Job drawing, mm, ordinate dimensions from the low corner. One solid piece. Coordinates: 2 decimals unless noted, no trailing zeros. Order: outer loops, then holes, each group sorted by start corner. A loop starts at its lowest first (then second) coordinate and runs counter-clockwise, first axis right, second up. Notation, with made-up numbers: (81, 69) - (127, 69) arc R19 ccw to (127, 89) - close; hole circle Ø1 at (35, 65.25). An arc over 180 degrees is marked (long way). Return JSON: item names as keys, results as strings.
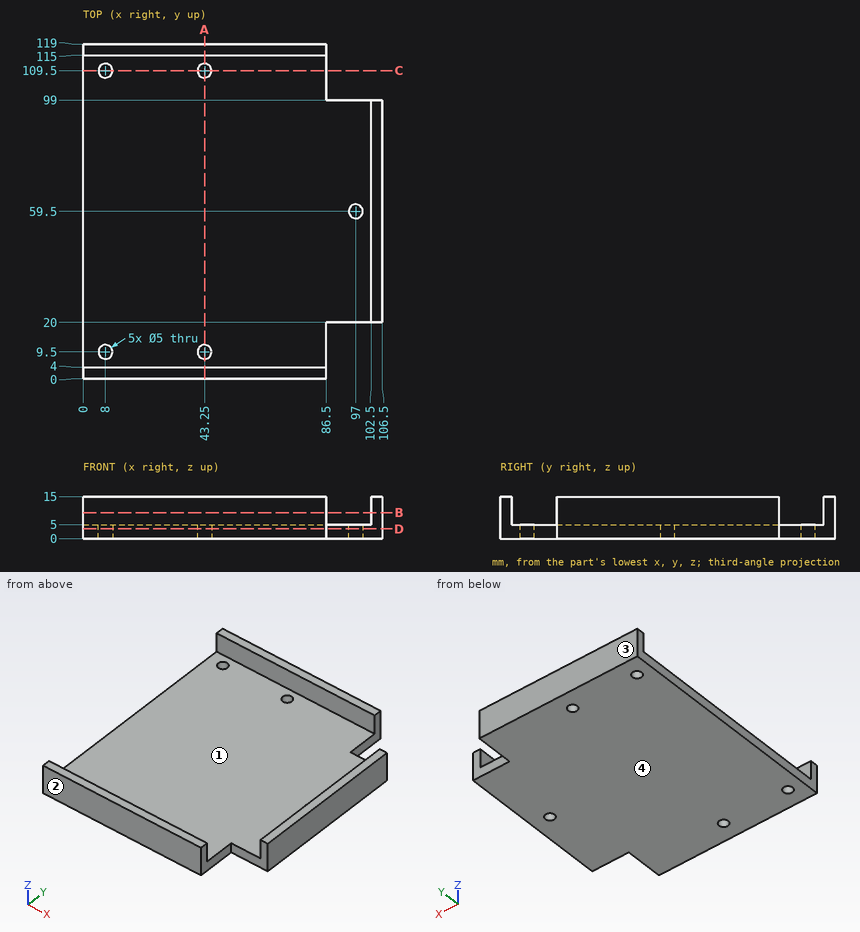
1. Cut at B-B on z = 9.25. Give the cut face in (x, y), plus the area to 3 significant figures.
Check values:
{"outline": "(0, 0) - (86.5, 0) - (86.5, 4) - (0, 4) - close; (0, 115) - (86.5, 115) - (86.5, 119) - (0, 119) - close; (102.5, 20) - (106.5, 20) - (106.5, 99) - (102.5, 99) - close", "area": "1,010 mm²"}
2. Cut at D-D on z = 3.5. Give the cut face in (x, y), plus the area to 3 significant figures.
Check values:
{"outline": "(0, 0) - (86.5, 0) - (86.5, 20) - (106.5, 20) - (106.5, 99) - (86.5, 99) - (86.5, 119) - (0, 119) - close; hole circle Ø5 at (8, 9.5); hole circle Ø5 at (8, 109.5); hole circle Ø5 at (43.25, 9.5); hole circle Ø5 at (43.25, 109.5); hole circle Ø5 at (97, 59.5)", "area": "11,800 mm²"}
3. Drop flat-ended pins along their axis: pin 1 (12 mm diameter, centred on x = 17.5, y = 106.5, fed in from +Z); pin 2 (3 mm diameter, centred on x = 79.5, z = 8.5, fed in from -Y); pin 3 (7.5 mm diameter, centred on x = 99, z = 10.5, fed in from -Y); pin 4 (5 mm diameter, centred on y = 63, z = 10, fed in from -X). Give the stop position or say it passes through.
Check values:
{"pin 1": "z = 5", "pin 2": "y = 0", "pin 3": "y = 20", "pin 4": "x = 102.5"}
4. Probe L1, parallel to Y at x = 8, z = 2.95; L2, parallel to Y at x = 65.5, z = 8; L3, parallel to Y at x = 97, z = 3. List the from-to ranges inside material, lowest first.
Check values:
{"L1": "0 to 7, 12 to 107, 112 to 119", "L2": "0 to 4, 115 to 119", "L3": "20 to 57, 62 to 99"}
5. Cut at A-A on x = 43.25. Give the cut face in (y, z), plus the area to 3 significant figures.
Check values:
{"outline": "(0, 0) - (7, 0) - (7, 5) - (4, 5) - (4, 15) - (0, 15) - close; (12, 0) - (107, 0) - (107, 5) - (12, 5) - close; (112, 0) - (119, 0) - (119, 15) - (115, 15) - (115, 5) - (112, 5) - close", "area": "625 mm²"}
6. Mould opens along Y. For the marked faces 1, 2, 3 and 4 say: pulls with the +Y half, pulls with the -Y half, needs draft (parallel to the pull), parting line crosses it, or undercut.
Check values:
{"face 1": "undercut", "face 2": "pulls with the -Y half", "face 3": "pulls with the +Y half", "face 4": "needs draft"}
7. Cut at C-C on y = 109.5. Give the cut face in (x, z).
Check values:
{"outline": "(0, 0) - (5.5, 0) - (5.5, 5) - (0, 5) - close; (10.5, 0) - (40.75, 0) - (40.75, 5) - (10.5, 5) - close; (45.75, 0) - (86.5, 0) - (86.5, 5) - (45.75, 5) - close"}
